The model under review builds one solid part; all positions refer to its coordinate system, in mm. Face numbers are marked on the shaded views. A direction names the side the tool comes from. Give positions to 0.01 mm unless a question says otherwise; leave off trailing zeros. Loops run counter-clockwise (first coordinate to the right, second up) from the corner with the lowest first, then second, coordinate; pieces in that order, holes last. Notation, with made-up numbers: M -6,61 L 22,61 A30 cw 22,90 Z; hole C 43.25,27 d7. An arc over 180 degrees is marked long. Put each result on its own line as item: value. Start each with the question number.
```python
from build123d import *

# Parameters (mm, degrees)
ESTRUSIONE_ESTRUSIONE2_DEPTH                         = 30
FORO_LAMATO_PER_VITE_M4_A_TESTA_CILINDRI_D           = 4.5
FORO_LAMATO_PER_VITE_M4_A_TESTA_CILINDRI_DEPTH       = 15
FORO_LAMATO_PER_VITE_M4_A_TESTA_CILINDRI_CBORE_D     = 10
FORO_LAMATO_PER_VITE_M4_A_TESTA_CILINDRI_CBORE_DEPTH = 3.5
FORO_LAMATO_PER_VITE_M4_A_TESTA_CILINDRI_TIP         = 1.351936393
SCHIZZO6_R                                           = 10
TAGLIO_ESTRUSIONE1_DEPTH                             = 2


with BuildPart() as part:
    # Schizzo2 → Estrusione-Estrusione2 (new body)
    with BuildSketch(Plane(origin=(0, 0, 0), x_dir=(1, 0, 0), z_dir=(0, 1, 0))):
        Polygon((0, 25), (0, 0), (10, -10), (35, -10), (35, -15), (-5, -15), (-5, 25), align=None)
    extrude(amount=ESTRUSIONE_ESTRUSIONE2_DEPTH)

    # Foro lamato per Vite M4 a testa cilindrica piana-1
    with Locations(Plane(origin=(0, 0, 0), x_dir=(0, 0, -1), z_dir=(1, 0, 0))):
        with Locations((12.5, 15)):
            CounterBoreHole(FORO_LAMATO_PER_VITE_M4_A_TESTA_CILINDRI_D / 2, FORO_LAMATO_PER_VITE_M4_A_TESTA_CILINDRI_CBORE_D / 2, FORO_LAMATO_PER_VITE_M4_A_TESTA_CILINDRI_CBORE_DEPTH, depth=FORO_LAMATO_PER_VITE_M4_A_TESTA_CILINDRI_DEPTH)
            with Locations((0, 0, -(FORO_LAMATO_PER_VITE_M4_A_TESTA_CILINDRI_DEPTH + FORO_LAMATO_PER_VITE_M4_A_TESTA_CILINDRI_TIP / 2))):  # 118° drill point
                Cone(0, FORO_LAMATO_PER_VITE_M4_A_TESTA_CILINDRI_D / 2, FORO_LAMATO_PER_VITE_M4_A_TESTA_CILINDRI_TIP, mode=Mode.SUBTRACT)

    # Schizzo6 → Taglio-Estrusione1 (cut)
    with BuildSketch(Plane.XY.offset(15)):
        with Locations((15, 15)):
            Circle(SCHIZZO6_R)
    extrude(amount=-TAGLIO_ESTRUSIONE1_DEPTH, mode=Mode.SUBTRACT)


solid = part.part
```
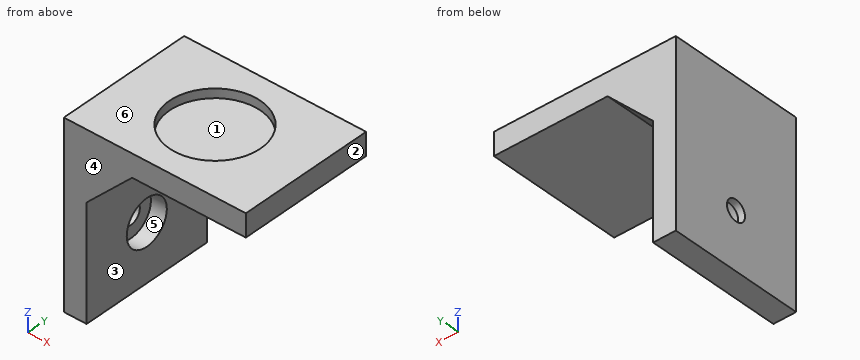
Item 1: Tool access review of the marked faces 1, 2 and 3: name each direction out of +Z, -Z, +X, -X, +Y, -Y from which nothing blocks a thin tool from reaching the whole face with its end or side.
Item 2: Consider section C-C, the plane x = 15. Write out the cut boundary in (y, z), plus the area to 3 significant figures.
Item 3: Clearance check with flat-ended pins moving along their axes: pin 1 Ø5 at (y, z) = (27, -14) entering from +X; pin 2 Ø6 at (y, z) = (15, -12.5) entering from +X; pin 3 Ø10 at (x, y) = (14.5, 12) entering from +Z; pin 4 Ø3 at (x, z) = (2.5, 11) entering from -Y. State where each tip first meets the part, or that it passes through.
Item 4: Draft analysis for pull direction Y (two halves, no side actions). For the marked faces 4, 5 and 6, state which applies: +Y half, -Y half, draft (parallel to the pull), parting line (faces both ways), or undercut.
Item 5: To check wall thickness, follow L1, parallel to Y at x = 15, z = 14.45; L2, parallel to Y at x = -0.95, z = -12.5; L3, parallel to Z at x = 11, y = 26. State the ranges of each line that lie inside material, in increasing order. Write a range as [from, to].
Item 6: Consider section D-D, the plane y = 28. Write out the cut boundary in (x, z).
Item 7: Consider section A-A, the plane z = -12.5. Write out the cut boundary in (x, y), plus the area to 3 significant figures.
Item 8: Consider section B-B, the plane y = 15. Write out the cut boundary in (x, z), plus the area to 3 significant figures.
Report:
1. face 1: +Z
1. face 2: +Z, -Z, +X, +Y, -Y
1. face 3: -Z, +X, +Y, -Y
2. outline: M 0,10 L 30,10 L 30,15 L 25,15 L 25,13 L 5,13 L 5,15 L 0,15 Z
2. area: 110 mm²
3. pin 1: x = 0
3. pin 2: x = -3.5
3. pin 3: z = 13
3. pin 4: y = 0
4. face 4: -Y half
4. face 5: undercut
4. face 6: draft
5. L1: [0, 5], [25, 30]
5. L2: [0, 10], [20, 30]
5. L3: [10, 15]
6. outline: M -5,-25 L 0,-25 L 0,0 L 10,10 L 35,10 L 35,15 L -5,15 Z
7. outline: M -5,0 L 0,0 L 0,10 L -3.5,10 L -3.5,12.75 L -5,12.75 Z; M -5,17.25 L -3.5,17.25 L -3.5,20 L 0,20 L 0,30 L -5,30 Z
7. area: 108 mm²
8. outline: M -5,-25 L 0,-25 L 0,-17.5 L -3.5,-17.5 L -3.5,-14.75 L -5,-14.75 Z; M -5,-10.25 L -3.5,-10.25 L -3.5,-7.5 L 0,-7.5 L 0,0 L 10,10 L 35,10 L 35,15 L 25,15 L 25,13 L 5,13 L 5,15 L -5,15 Z
8. area: 343 mm²
